Read the model definition and answer for the solid it produces. Units are mm, in the model's axes. Face numbers are marked on the shaded views. Round coordinates to 2 decimals unless told otherwise and drop trailing zeros. Order: outer loops, then holes, each group sorted by start corner. A loop starts at its lowest first (then second) coordinate and runs counter-clockwise, first axis right, second up.
from build123d import *

# Parameters (mm, degrees)
SKETCH1_W           = 200
SKETCH1_H           = 400
SKETCH1_R           = 15
SKETCH1_R_2         = 5
BOSS_EXTRUDE1_DEPTH = 7.5
SKETCH4_W           = 11
SKETCH4_H           = 400
BOSS_EXTRUDE4_DEPTH = 72.5
SKETCH5_R           = 4
CUT_EXTRUDE1_DEPTH  = 200
SKETCH6_R           = 3
CUT_EXTRUDE2_DEPTH  = 10


with BuildPart() as part:
    # Sketch1 → Boss-Extrude1 (new body)
    with BuildSketch(Plane.XY):
        Rectangle(SKETCH1_W, SKETCH1_H)
        with Locations((0, -125)):
            Circle(SKETCH1_R, mode=Mode.SUBTRACT)
        with Locations((-65, 0)):
            Circle(SKETCH1_R_2, mode=Mode.SUBTRACT)
        with Locations((-65, 100)):
            Circle(SKETCH1_R_2, mode=Mode.SUBTRACT)
        with Locations((65, 100)):
            Circle(SKETCH1_R_2, mode=Mode.SUBTRACT)
        with Locations((65, 0)):
            Circle(SKETCH1_R_2, mode=Mode.SUBTRACT)
    extrude(amount=BOSS_EXTRUDE1_DEPTH)

    # Sketch4 → Boss-Extrude4 (add)
    with BuildSketch(Plane.XY.offset(7.5)):
        with Locations((-94.5, 0)):
            Rectangle(SKETCH4_W, SKETCH4_H)
        with Locations((94.5, 0)):
            Rectangle(SKETCH4_W, SKETCH4_H)
    extrude(amount=BOSS_EXTRUDE4_DEPTH)

    # Sketch5 → Cut-Extrude1 (cut)
    with BuildSketch(Plane(origin=(100, 0, 0), x_dir=(0, 0, -1), z_dir=(1, 0, 0))):
        with Locations((-58, 100)):
            Circle(SKETCH5_R)
        with Locations((-58, 0)):
            Circle(SKETCH5_R)
        with Locations((-58, -100)):
            Circle(SKETCH5_R)
    extrude(amount=-CUT_EXTRUDE1_DEPTH, mode=Mode.SUBTRACT)

    # Sketch6 → Cut-Extrude2 (cut)
    with BuildSketch(Plane.XY):
        with Locations((31.797314882, -93.202685118)):
            Circle(SKETCH6_R)
        with Locations((-31.797314882, -93.202685118)):
            Circle(SKETCH6_R)
        with Locations((-31.797314882, -156.797314882)):
            Circle(SKETCH6_R)
        with Locations((31.797314882, -156.797314882)):
            Circle(SKETCH6_R)
    extrude(amount=CUT_EXTRUDE2_DEPTH, mode=Mode.SUBTRACT)


solid = part.part
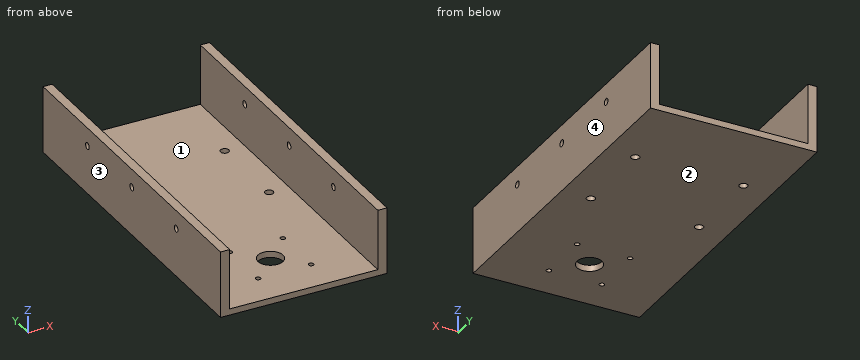
Q1. A cutting plane is placed at D-D, the plane y = -125. Give the vertices of the cut face in (x, z), plus the area to 3 significant figures.
Outcome:
outline: (-100, 0) - (-15, 0) - (-15, 7.5) - (-89, 7.5) - (-89, 80) - (-100, 80) - close; (15, 0) - (100, 0) - (100, 80) - (89, 80) - (89, 7.5) - (15, 7.5) - close
area: 2,870 mm2
Q2. For a pull along X with two mould halves and no side action, classify the marked faces 1, 2, 3 and 4 as released by +X, released by -X, zero draft, split by the parting line, or undercut.
Outcome:
face 1: undercut
face 2: zero draft
face 3: released by -X
face 4: released by +X
Q3. A cutting plane is placed at C-C, the plane x = 0. Give the vertices of the cut face in (y, z).
Outcome:
outline: (-200, 0) - (-140, 0) - (-140, 7.5) - (-200, 7.5) - close; (-110, 0) - (200, 0) - (200, 7.5) - (-110, 7.5) - close
Q4. A cutting plane is placed at A-A, the plane y = 100. Give the vertices of the cut face in (x, z), plus the area to 3 significant figures.
Outcome:
outline: (-100, 0) - (-70, 0) - (-70, 7.5) - (-89, 7.5) - (-89, 54) - (-100, 54) - close; (-100, 62) - (-89, 62) - (-89, 80) - (-100, 80) - close; (-60, 0) - (60, 0) - (60, 7.5) - (-60, 7.5) - close; (70, 0) - (100, 0) - (100, 54) - (89, 54) - (89, 7.5) - (70, 7.5) - close; (89, 62) - (100, 62) - (100, 80) - (89, 80) - close
area: 2,770 mm2
Q5. A cutting plane is placed at B-B, the plane z = 48.5. Give the vertices of the cut face in (x, y), plus the area to 3 significant figures.
Outcome:
outline: (-100, -200) - (-89, -200) - (-89, 200) - (-100, 200) - close; (89, -200) - (100, -200) - (100, 200) - (89, 200) - close
area: 8,800 mm2
Q6. Straight lines are drawn through the part: probe 1 along Y at (x, z) = (94, 58); probe 2 along Y at (x, z) = (-65, 4.5); probe 3 along X at (y, z) = (104, 57). For each, find the intervals that lie inside material, in ascending order.
Outcome:
probe 1: y = -200 to -104, -96 to -4, 4 to 96, 104 to 200
probe 2: y = -200 to -5, 5 to 95, 105 to 200
probe 3: x = -100 to -89, 89 to 100
Q7. A flat-ended cylindrical pin translates along its axis: pin 1 (3.5 mm diameter, centred on x = -31.8, y = -93.2, fed in from -Z) (3 decimals). Find the tip coordinate at first contact, or state that the pin passes through.
Outcome:
pin 1: passes through
